Solid Edge part; units mm, degrees
sketch "Sketch1" plane through (0, 0, 0) normal (0, 0, 1) x (1, 0, 0)
  line L0 (-4, 42.5) -> (-4, -42.5)
  line L1 (-4, -42.5) -> (4, -42.5)
  line L2 (4, -42.5) -> (4, 42.5)
  line L3 (4, 42.5) -> (-4, 42.5)
extrude "Protrusion1" add sketch "Sketch1" along normal mid plane 10
fillet "Round_2" radius 2 4 edges at (-4, 0, 5) (4, 0, 5) (-4, 0, -5) (4, 0, -5)
fillet "Round_3" radius 2 14 edges at (-3.4142, 42.5, 4.4142) (0, 42.5, 5) (3.4142, 42.5, 4.4142) (4, 42.5, 0) (0, 42.5, -5) (-3.4142, 42.5, -4.4142) (-4, 42.5, 0) (0, -42.5, 5) (-3.4142, -42.5, 4.4142) (-4, -42.5, 0) (-3.4142, -42.5, -4.4142) (0, -42.5, -5) (3.4142, -42.5, -4.4142) (4, -42.5, 0)
sketch "Sketch2" plane through (0, 0, 0) normal (0, 0, 1) x (1, 0, 0)
  circle A0 centre (9, -18.5) radius 3.2
  line L0 (14, -13.5) -> (14, -23.5)
  line L1 (14, -23.5) -> (4, -23.5)
  line L2 (4, -23.5) -> (4, -13.5)
  line L3 (4, -13.5) -> (14, -13.5)
extrude "ExtrudedProtrusion_4" add sketch "Sketch2" against normal blind 2.5
fillet "Round_5" radius 3 4 edges at (14, -13.5, -1.25) (14, -23.5, -1.25) (4, -13.5, -1.25) (4, -23.5, -1.25)
sketch "Sketch3" plane through (0, 0, 0) normal (0, 0, 1) x (1, 0, 0)
  circle A0 centre (0, 36.5) radius 2.5
extrude "ExtrudedCutout_2" cut sketch "Sketch3" along normal mid plane 10
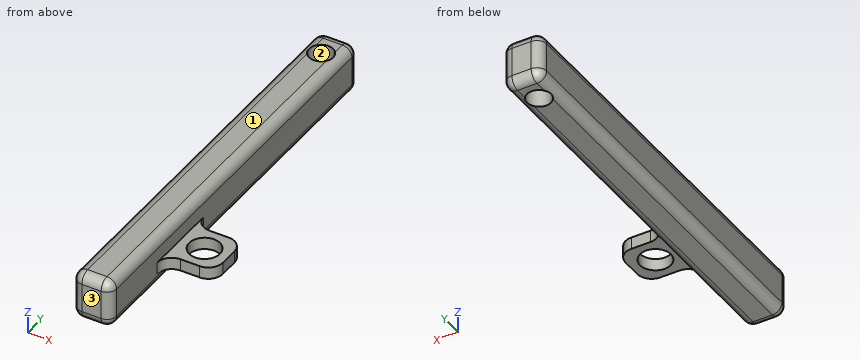
Design review of the part built by this model. Coordinates are the model's own, in mm. Face numbers are marked on the shaded views. Coordinates: 2 decimals unless noted, no trailing zeros. Order: outer loops, then holes, each group sorted by start corner. A loop starts at its lowest first (then second) coordinate and runs counter-clockwise, first axis right, second up. Notation, with made-up numbers: (55, 9.5) - (84, 9.5) arc R9 ccw to (84, 26.5) - close; hole circle Ø2 at (44, 52.5). An arc over 180 degrees is marked (long way). One line per question, with ' | ' between items.
Q1. Consider section A-A, the plane x = 0. Give the boundary of the cut face in (y, z).
Answer key:
outline: (-42.5, -3) arc R2 ccw to (-40.5, -5) - (34, -5) - (34, 5) - (-40.5, 5) arc R2 ccw to (-42.5, 3) - close; (39, -5) - (40.5, -5) arc R2 ccw to (42.5, -3) - (42.5, 3) arc R2 ccw to (40.5, 5) - (39, 5) - close
Q2. Consider section C-C, the plane z = -4. Give the boundary of the cut face in (x, y), then the cut area to 3 significant figures.
Answer key:
outline: (-3.73, -40.5) arc R1.73 ccw to (-2, -42.23) - (2, -42.23) arc R1.73 ccw to (3.73, -40.5) - (3.73, 40.5) arc R1.73 ccw to (2, 42.23) - (-2, 42.23) arc R1.73 ccw to (-3.73, 40.5) - close; hole circle Ø5 at (0, 36.5) | area: 608 mm2
Q3. Consider section B-B, the plane y = -18.5. Give the boundary of the cut face in (x, z), then the cut area to 3 significant figures.
Answer key:
outline: (-4, -3) arc R2 ccw to (-2, -5) - (2, -5) arc R2 ccw to (4, -3) - (4, -2.5) - (5.8, -2.5) - (5.8, 0) - (4, 0) - (4, 3) arc R2 ccw to (2, 5) - (-2, 5) arc R2 ccw to (-4, 3) - close; (12.2, -2.5) - (14, -2.5) - (14, 0) - (12.2, 0) - close | area: 85.6 mm2
Q4. To check wall thickness, follow line 1 along X through (y, z) = (36.5, 1.5); line 2 along Y through (x, z) = (9, -1.2); line 3 along X through (y, z) = (30, -3). State the ranges of each line that lie inside material, in increasing order.
Answer key:
line 1: x = -4 to -2.5, 2.5 to 4 | line 2: y = -23.5 to -21.7, -15.3 to -13.5 | line 3: x = -4 to 4
Q5. Clearance check with flat-ended pins moving along their axes: pin 1 Ø3 at (x, y) = (9, -17.5) entering from -Z; pin 2 Ø6 at (y, z) = (5, -2) entering from +X; pin 3 Ø5 at (x, y) = (11.5, -16) entering from +Z; pin 4 Ø1.2 at (x, z) = (8.5, -1) entering from +Y. State where each tip first meets the part, or that it passes through.
Answer key:
pin 1: passes through | pin 2: stops at x = 4 | pin 3: stops at z = 0 | pin 4: stops at y = -13.5
Q6. Consider section D-D, the plane y = -29. Give the boundary of the cut face in (x, z).
Answer key:
outline: (-4, -3) arc R2 ccw to (-2, -5) - (2, -5) arc R2 ccw to (4, -3) - (4, 3) arc R2 ccw to (2, 5) - (-2, 5) arc R2 ccw to (-4, 3) - close
Q7. The part is to be moulded in two halves that separate along Y. For the marked faces 1, 2 and 3, say which applies: +Y half, -Y half, draft (parallel to the pull), parting line (faces both ways), or undercut.
Answer key:
face 1: draft | face 2: undercut | face 3: -Y half
